from build123d import *

# Parameters (mm, degrees)
SKETCH2_W           = 100
SKETCH2_H           = 200
BOSS_EXTRUDE1_DEPTH = 55
SKETCH3_R           = 10
CUT_EXTRUDE1_DEPTH  = 110
SKETCH4_R           = 12.5
CUT_EXTRUDE2_DEPTH  = 100
FILLET1_R           = 10


with BuildPart() as part:
    # Sketch2 → Boss-Extrude1 (new body, symmetric)
    with BuildSketch(Plane.XY):
        Rectangle(SKETCH2_W, SKETCH2_H)
        with BuildLine():
            ThreePointArc((50, -150), (0, -200), (-50, -150))
            Line((-50, -150), (-50, -100))
            Line((-50, -100), (50, -100))
            Line((50, -100), (50, -150))
        make_face()
    extrude(amount=BOSS_EXTRUDE1_DEPTH, both=True)

    # Sketch3 → Cut-Extrude1 (cut)
    with BuildSketch(Plane.XY.offset(55)):
        with Locations((0, -150)):
            Circle(SKETCH3_R)
    extrude(amount=-CUT_EXTRUDE1_DEPTH, mode=Mode.SUBTRACT)

    # Sketch4 → Cut-Extrude2 (cut)
    with BuildSketch(Plane(origin=(0, 100, 0), x_dir=(1, 0, 0), z_dir=(0, 1, 0))):
        Circle(SKETCH4_R)
    extrude(amount=-CUT_EXTRUDE2_DEPTH, mode=Mode.SUBTRACT)

    # Fillet1
    fillet1_edges = [part.edges().sort_by_distance(p)[0] for p in [
        (50, 100, 0),
        (-50, -25, 55),
        (-10, -150, -55),
        (0, -200, 55),
        (50, -25, 55),
        (0, -200, -55),
        (-50, -25, -55),
        (0, 100, -55),
        (50, -25, -55),
        (-50, 100, 0),
    ]]
    fillet(fillet1_edges, radius=FILLET1_R)


solid = part.part
Geometry: final body of the model. Coordinates: model frame, mm. A direction names the side the tool comes from. Round coordinates to 2 decimals unless told otherwise and drop trailing zeros. Order: outer loops, then holes, each group sorted by start corner. A loop starts at its lowest first (then second) coordinate and runs counter-clockwise, first axis right, second up.
Q1. Section B-B, the plane z = 30.5. Output: boundary loops of the cut face in (x, y), and give its area (3 significant figures).
Result sheet:
outline: (-50, -150) arc R50 ccw to (50, -150) - (50, 90) arc R10 ccw to (40, 100) - (-40, 100) arc R10 ccw to (-50, 90) - close; hole circle Ø20 at (0, -150)
area: 28,600 mm2
Q2. Pin query (flat end, axial travel): pin 1 (1.5 mm diameter, centred on x = 38, z = -1.5, fed in from -Y); pin 2 (1.5 mm diameter, centred on x = 39, z = 15.5, fed in from -Y); pin 3 (1 mm diameter, centred on x = 19.5, z = 38, fed in from -Y). Return the tip coordinate at first contact, or that it passes through.
Result sheet:
pin 1: stops at y = -183.35
pin 2: stops at y = -182.2
pin 3: stops at y = -196.25
Q3. Section C-C, the plane z = 0. Output: boundary loops of the cut face in (x, y), and give its area (3 significant figures).
Result sheet:
outline: (-50, -150) arc R50 ccw to (50, -150) - (50, 90) arc R10 ccw to (40, 100) - (12.5, 100) - (12.5, 0) - (-12.5, 0) - (-12.5, 100) - (-40, 100) arc R10 ccw to (-50, 90) - close; hole circle Ø20 at (0, -150)
area: 26,100 mm2
Q4. Mould query, pull axis X, two halves, no side actions, for faces 3 (the face through (-47.15, 96.99, 4.3)), 4 (the face through (46.99, -31.68, -52.15)), 5 (the face through (11.923, 50.7, -3.755)), 6 (the face through (0.56, 96.99, -52.15)). Classes: released by +X, released by -X, zero draft, split by the parting line, or undercut.
Result sheet:
face 3: released by -X
face 4: released by +X
face 5: undercut
face 6: zero draft
Q5. Section A-A, the plane x = 0. Output: boundary loops of the cut face in (y, z), and give its area (3 significant figures).
Result sheet:
outline: (-200, -45) arc R10 ccw to (-190, -55) - (-170, -55) arc R10 ccw to (-160, -45) - (-160, 55) - (-190, 55) arc R10 ccw to (-200, 45) - close; (-140, -45) arc R10 ccw to (-130, -55) - (90, -55) arc R10 ccw to (100, -45) - (100, -12.5) - (0, -12.5) - (0, 12.5) - (100, 12.5) - (100, 55) - (-140, 55) - close
area: 28,200 mm2
Q6. Material intervals for probe 1 along X at (y, z) = (75.5, 0); probe 2 along Z at (x, y) = (0, 78); probe 3 along Y at (x, z) = (2, -18), sorted ascending.
Result sheet:
probe 1: x = -50 to -12.5, 12.5 to 50
probe 2: z = -55 to -12.5, 12.5 to 55
probe 3: y = -199.96 to -159.8, -140.2 to 100
Q7. Access query for faces 1 (the face through (0, 0, 0)), 2 (the face through (47.15, -23.25, 51.99)). Directions: +Z, -Z, +X, -X, +Y, -Y. A direction counts if a zero-diameter tool reaches every point of the face in a straight line with its end or side. Return the directions, or none.
Result sheet:
face 1: +Y
face 2: +Z, +X, +Y, -Y
